```python
from build123d import *

# Parameters (mm, degrees)
SKETCH1_W             = 38
SKETCH1_H             = 28
BOARD_DEPTH           = 1.6
PROBE_CONNECTOR_START = 1.6
SKETCH2_W             = 6
SKETCH2_H             = 10
PROBE_CONNECTOR_DEPTH = 6
SIGNAL_HEADER_START   = 1.6
SKETCH3_W             = 5
SKETCH3_H             = 8
SIGNAL_HEADER_DEPTH   = 6
TRIM_POT_START        = 1.6
SKETCH4_W             = 9.5
SKETCH4_H             = 9.5
TRIM_POT_DEPTH        = 5


with BuildPart() as part:
    # Sketch1 → Board (new body)
    with BuildSketch(Plane(origin=(0, 0, 0), x_dir=(1, 0, 0), z_dir=(0, 1, 0))):
        Rectangle(SKETCH1_W, SKETCH1_H)
    extrude(amount=BOARD_DEPTH)

    # Sketch2 → Probe_Connector (add)
    with BuildSketch(Plane(origin=(0, 0, 0), x_dir=(1, 0, 0), z_dir=(0, 1, 0)).offset(PROBE_CONNECTOR_START)):
        with Locations((-14, 0)):
            Rectangle(SKETCH2_W, SKETCH2_H)
    extrude(amount=PROBE_CONNECTOR_DEPTH)

    # Sketch3 → Signal_Header (add)
    with BuildSketch(Plane(origin=(0, 0, 0), x_dir=(1, 0, 0), z_dir=(0, 1, 0)).offset(SIGNAL_HEADER_START)):
        with Locations((15, 0)):
            Rectangle(SKETCH3_W, SKETCH3_H)
    extrude(amount=SIGNAL_HEADER_DEPTH)

    # Sketch4 → Trim_Pot (add)
    with BuildSketch(Plane(origin=(0, 0, 0), x_dir=(1, 0, 0), z_dir=(0, 1, 0)).offset(TRIM_POT_START)):
        with Locations((2, 0)):
            Rectangle(SKETCH4_W, SKETCH4_H)
    extrude(amount=TRIM_POT_DEPTH)


solid = part.part
```
Check sheet for the modelled part. Datum: model origin and axes. Units: mm. A direction names the side the tool comes from. Round coordinates to 2 decimals unless told otherwise and drop trailing zeros. Order: outer loops, then holes, each group sorted by start corner. A loop starts at its lowest first (then second) coordinate and runs counter-clockwise, first axis right, second up. Notation, with made-up numbers: M 60.5,83.5 L 72.5,83.5 A11 cw 72.5,96.5 Z; hole C 2,-12 d1. An arc over 180 degrees is marked long. Answer in a Markdown table with one row per item.
(1) Section check C-C on z = 8.75. Record the boundary of the cut face in (x, y).
Findings:
| item | result |
|---|---|
| outline | M -19,0 L 19,0 L 19,1.6 L -19,1.6 Z |
(2) Section check B-B on x = -16. Record the boundary of the cut face in (y, z).
Findings:
| item | result |
|---|---|
| outline | M 0,-14 L 1.6,-14 L 1.6,-5 L 7.6,-5 L 7.6,5 L 1.6,5 L 1.6,14 L 0,14 Z |
(3) Set-up check for faces 5 (the flat face through (-14, 5, -5)), 6 (the flat face through (12.5, 5, 0)), 7 (the flat face through (-14, 5, 5)): record each of +Z, -Z, +X, -X, +Y, -Y from which the full face is reachable in a straight line by a thin tool's end or side.
Findings:
| item | result |
|---|---|
| face 5 | -Z, +X, -X, +Y |
| face 6 | +Z, -Z, +Y |
| face 7 | +Z, +X, -X, +Y |
(4) Draft check along X on faces 1 (the flat face through (-19, 1, 0)), 2 (the flat face through (0, 0, 0)), 3 (the flat face through (17.5, 5, 0)), 4 (the flat face through (6.75, 4, 0)). Enter one of: +X half, -X half, draft (parallel to the pull), parting line (faces both ways), or undercut.
Findings:
| item | result |
|---|---|
| face 1 | -X half |
| face 2 | draft |
| face 3 | +X half |
| face 4 | undercut |
(5) Section check D-D on x = 15.5. Record the boundary of the cut face in (y, z), plus the area to 3 significant figures.
Findings:
| item | result |
|---|---|
| outline | M 0,-14 L 1.6,-14 L 1.6,-4 L 7.6,-4 L 7.6,4 L 1.6,4 L 1.6,14 L 0,14 Z |
| area | 92.8 mm^2 |
(6) Gauge pin test, flat ends, axial feed: pin 1 (6 mm diameter, centred on x = 7, z = -7, fed in from +Y); pin 2 (1.5 mm diameter, centred on x = -4, y = 5, fed in from +Z); pin 3 (4 mm diameter, centred on x = 1.5, y = 4.5, fed in from -Z); pin 4 (1.5 mm diameter, centred on y = 5, z = 1.5, fed in from -X). Record the tip position at first contact, or that the pin passes through.
Findings:
| item | result |
|---|---|
| pin 1 | stops at y = 6.6 |
| pin 2 | passes through |
| pin 3 | stops at z = -4.75 |
| pin 4 | stops at x = -17 |
(7) Material ranges on line 1 along X through (y, z) = (4, -1); line 2 along Y through (x, z) = (-4, -6.75); line 3 along Y through (x, z) = (4, -4), recorded low to high. Write a range as from..to.
Findings:
| item | result |
|---|---|
| line 1 | x = -17..-11, -2.75..6.75, 12.5..17.5 |
| line 2 | y = 0..1.6 |
| line 3 | y = 0..6.6 |
(8) Section check A-A on y = 2. Record the boundary of the cut face in (x, z).
Findings:
| item | result |
|---|---|
| outline | M -17,-5 L -11,-5 L -11,5 L -17,5 Z; M -2.75,-4.75 L 6.75,-4.75 L 6.75,4.75 L -2.75,4.75 Z; M 12.5,-4 L 17.5,-4 L 17.5,4 L 12.5,4 Z |
